from build123d import *

# Parameters (mm, degrees)
SKETCH1_W               = 28.575
SKETCH1_H               = 7.9375
SKETCH1_R               = 2.4892
BOSS_EXTRUDE1_DEPTH     = 3.175
CUT_EXTRUDE1_DEPTH      = 16.164572457
CUT_EXTRUDE1_DEPTH_BACK = 16.164572457
SKETCH2_R               = 2.4892


with BuildPart() as part:
    # Sketch1 → Boss-Extrude1 (new, symmetric)
    with BuildSketch(Plane.XY):
        Rectangle(SKETCH1_W, SKETCH1_H)
        with Locations((-3.175, 0)):
            Circle(SKETCH1_R, mode=Mode.SUBTRACT)
        with Locations((9.525, 0)):
            Circle(SKETCH1_R, mode=Mode.SUBTRACT)
    extrude(amount=BOSS_EXTRUDE1_DEPTH, both=True)

    # Sketch2 → Cut-Extrude1 (cut, two sides: drawn at the far end of the back side and taken through both)
    with BuildSketch(Plane(origin=(0, 0, 0), x_dir=(1, 0, 0), z_dir=(0, 1, 0)).offset(-CUT_EXTRUDE1_DEPTH_BACK)):
        with Locations(Location((3.175, 0, 0), (0, 0, 270))):
            Circle(SKETCH2_R)
        with Locations(Location((-9.525, 0, 0), (0, 0, 270))):
            Circle(SKETCH2_R)
    extrude(amount=CUT_EXTRUDE1_DEPTH + CUT_EXTRUDE1_DEPTH_BACK, mode=Mode.SUBTRACT)


solid = part.part
Geometry check sheet. Reference: the model listing, model coordinates, mm. Give positions to 0.01 mm unless a question says otherwise; leave off trailing zeros. Order: outer loops, then holes, each group sorted by start corner. A loop starts at its lowest first (then second) coordinate and runs counter-clockwise, first axis right, second up.
1. Sectioned sample at D-D (y = 3). Record the boundary of the cut face in (x, z) (1 decimal).
Completed:
outline: (-14.3, -3.2) - (14.3, -3.2) - (14.3, 3.2) - (-14.3, 3.2) - close; hole circle Ø5 at (-9.5, 0); hole circle Ø5 at (3.2, 0)
2. Sectioned sample at C-C (x = 10). Record the boundary of the cut face in (y, z) (3 decimals), then the cut area to 3 significant figures.
Completed:
outline: (-3.969, -3.175) - (-2.443, -3.175) - (-2.443, 3.175) - (-3.969, 3.175) - close; (2.443, -3.175) - (3.969, -3.175) - (3.969, 3.175) - (2.443, 3.175) - close
area: 19.4 mm2
3. Sectioned sample at B-B (y = -1.75). Record the boundary of the cut face in (x, z) (1 decimal), then the cut area to 3 significant figures.
Completed:
outline: (-14.3, -3.2) - (-4.9, -3.2) - (-4.9, 3.2) - (-14.3, 3.2) - close; (-1.4, -3.2) - (7.8, -3.2) - (7.8, 3.2) - (-1.4, 3.2) - close; (11.3, -3.2) - (14.3, -3.2) - (14.3, 3.2) - (11.3, 3.2) - close; hole circle Ø5 at (-9.5, 0); hole circle Ø5 at (3.2, 0)
area: 97.6 mm2
4. Draft check along X on faces 1 (the face through (-5.66, 0.11, -0.04)), 2 (the face through (0, 3.969, 0)), 3 (the face through (14.288, 0, 0)), 4 (the face through (11.9, 0.75, -0.04)). Enter one of: pulls with the +X half, pulls with the -X half, needs draft (parallel to the pull), parting line crosses it, or undercut.
Completed:
face 1: undercut
face 2: needs draft
face 3: pulls with the +X half
face 4: undercut
5. Sectioned sample at A-A (z = -1). Record the boundary of the cut face in (x, y) (1 decimal).
Completed:
outline: (-14.3, -4) - (-11.8, -4) - (-11.8, 4) - (-14.3, 4) - close; (-7.2, -4) - (0.9, -4) - (0.9, 4) - (-7.2, 4) - close; (5.5, -4) - (14.3, -4) - (14.3, 4) - (5.5, 4) - close; hole circle Ø5 at (-3.2, 0); hole circle Ø5 at (9.5, 0)
6. Scan lines: line 1 (Y direction, x = -3.25, z = 2.25); line 2 (X direction, y = 1.75, z = -1.25); line 3 (X direction, y = -1, z = 1.5). Record each from-to range of solid material in increasing order.
Completed:
line 1: y = -3.97 to -2.49, 2.49 to 3.97
line 2: x = -14.29 to -11.68, -7.37 to -4.95, -1.4 to 1.02, 5.33 to 7.75, 11.3 to 14.29
line 3: x = -14.29 to -11.51, -7.54 to -5.45, -0.9 to 1.19, 5.16 to 7.25, 11.8 to 14.29
7. Depth check by flat-ended pin: pin 1 (4 mm diameter, centred on x = 9.525, y = 0, fed in from +Z). Enter the tip coordinate at first touch or a pass-through.
Completed:
pin 1: passes through
